For this review, take the finished solid that the model builds, in its own axes (mm). A direction names the side the tool comes from. Give positions to 0.01 mm unless a question says otherwise; leave off trailing zeros. Order: outer loops, then holes, each group sorted by start corner. A loop starts at its lowest first (then second) coordinate and runs counter-clockwise, first axis right, second up. Notation, with made-up numbers: M 85.5,33 L 114.5,33 A22 ccw 114.5,40 Z; hole C -3,75 d7. An arc over 180 degrees is marked long. Answer as CSV lines item,"result". Start each with the question number.
1. We need section B-B, the plane x = 25. Give the boundary of the cut face in (y, z).
2. Mouldability with a two-part tool opening along Y and no side actions: class faces 1 (the cylindrical face through (10, 0, 3)), 2 (the flat face through (-11, -6, 2)), 3 (the flat face through (-9, 0, 0)) as pulls with the +Y half, pulls with the -Y half, needs draft (parallel to the pull), parting line crosses it, or undercut.
3. Clearance check with a flat-ended pin moving along its axis: P1, Ø6.5, axis at x = 14, y = 0, coming from the +Z side. State where the tip first meets the part, or that it passes through.
4. Machinability: for faces 4 (the flat face through (14, 0, 2)), 5 (the flat face through (-11, 6, 2)), which of the approach directions +Z, -Z, +X, -X, +Y, -Y give a long, thin tool a straight path to every point of the face, cutting with its end or side? Answer none if there is none.
5. We need section A-A, the plane z = 2.7. Give the boundary of the cut face in (x, y).
6. For line 1 along Y through (x, z) = (25, 3.55); line 2 along Y through (x, z) = (-43.5, 0.8); line 3 along X through (y, z) = (-1.5, 2.8), list the stretches that pass through material, from the lowest coordinate up.
7. We need section C-C, the plane y = 0. Give the boundary of the cut face in (x, z), and give its area (3 significant figures).
8. We need section D-D, the plane x = 14. Give the boundary of the cut face in (y, z), and give its area (3 significant figures).
from build123d import *

# Parameters (mm, degrees)
SKETCH1_W           = 80
SKETCH1_H           = 12
SKETCH1_R           = 4
SKETCH1_R_2         = 2
BOSS_EXTRUDE1_DEPTH = 5
SKETCH2_R           = 4
BOSS_EXTRUDE2_DEPTH = 2


with BuildPart() as part:
    # Sketch1 → Boss-Extrude1 (new body)
    with BuildSketch(Plane.XY):
        with Locations((-10, 0)):
            Rectangle(SKETCH1_W, SKETCH1_H)
        with Locations((-34, 0)):
            Circle(SKETCH1_R, mode=Mode.SUBTRACT)
        with Locations((14, 0)):
            Circle(SKETCH1_R, mode=Mode.SUBTRACT)
        with Locations((-45, 0)):
            Circle(SKETCH1_R_2, mode=Mode.SUBTRACT)
        with Locations((25, 0)):
            Circle(SKETCH1_R_2, mode=Mode.SUBTRACT)
    extrude(amount=BOSS_EXTRUDE1_DEPTH)

    # Sketch2 → Boss-Extrude2 (add)
    with BuildSketch(Plane(origin=(0, 0, 0), x_dir=(-1, 0, 0), z_dir=(0, 0, -1))):
        with Locations((34, 0)):
            Circle(SKETCH2_R)
        with Locations((-14, 0)):
            Circle(SKETCH2_R)
    extrude(amount=-BOSS_EXTRUDE2_DEPTH)


solid = part.part
Result set:
1,outline,"M -6,0 L -2,0 L -2,5 L -6,5 Z; M 2,0 L 6,0 L 6,5 L 2,5 Z"
2,face 1,"undercut"
2,face 2,"pulls with the -Y half"
2,face 3,"needs draft"
3,P1,"z = 2"
4,face 4,"+Z"
4,face 5,"+Z, -Z, +X, -X, +Y"
5,outline,"M -50,-6 L 30,-6 L 30,6 L -50,6 Z; hole C -45,0 d4; hole C -34,0 d8; hole C 14,0 d8; hole C 25,0 d4"
6,line 1,"-6 to -2, 2 to 6"
6,line 2,"-6 to -1.32, 1.32 to 6"
6,line 3,"-50 to -46.32, -43.68 to -37.71, -30.29 to 10.29, 17.71 to 23.68, 26.32 to 30"
7,outline,"M -50,0 L -47,0 L -47,5 L -50,5 Z; M -43,0 L 23,0 L 23,5 L 18,5 L 18,2 L 10,2 L 10,5 L -30,5 L -30,2 L -38,2 L -38,5 L -43,5 Z; M 27,0 L 30,0 L 30,5 L 27,5 Z"
7,area,"312 mm2"
8,outline,"M -6,0 L 6,0 L 6,5 L 4,5 L 4,2 L -4,2 L -4,5 L -6,5 Z"
8,area,"36.0 mm2"
